Autodesk Inventor part; units mm, degrees
ref_plane "XZ Plane" through (0, 0, 0) normal (0, 1, 0) x (-1, 0, 0)
ref_plane "XY Plane" through (0, 0, 0) normal (0, 0, 1) x (1, 0, 0)
sketch "Sketch1" plane through (0, 0, 0) normal (0, 1, 0) x (-1, 0, 0)
  line L0 (63.5, 50.8) -> (-63.5, 50.8)
  line L1 (-63.5, 50.8) -> (-63.5, -50.8)
  line L2 (-63.5, -50.8) -> (63.5, -50.8)
  line L3 (63.5, -50.8) -> (63.5, 50.8)
  line L4 (63.5, 50.8) -> (-63.5, -50.8) construction
  line L5 (-63.5, 50.8) -> (63.5, -50.8) construction
  point P0 (0, 0)
  dimension "d3" = 101.6
  dimension "d13" = 127
extrude "Extrusion1" add sketch "Sketch1" against normal blind 6.35
sketch "Sketch3" plane through (0, 0, 0) normal (0, 1, 0) x (1, 0, 0)
  line L0 (-63.5, -50.8) -> (-63.5, 50.8) construction
  line L1 (-63.5, -25.4) -> (63.5, -25.4) construction
  line L2 (63.5, 50.8) -> (63.5, -50.8) construction
  line L3 (63.5, 50.8) -> (-63.5, 50.8) construction
  circle A0 centre (-50.8, -25.4) radius 6.35
  circle A1 centre (-25.4, -25.4) radius 6.35
  circle A2 centre (0, -25.4) radius 6.35
  circle A3 centre (25.4, -25.4) radius 6.35
  circle A4 centre (50.8, -25.4) radius 6.35
  point P0 (0, 0)
  dimension "d2" = 76.2
  dimension "d4" = 12.7
  dimension "d5" = 12.7
  dimension "d8" = 25.4
extrude "Extrusion2" cut sketch "Sketch3" against normal through all
properties part number "5-holes"
Geometry check sheet. Reference: the model listing, model coordinates, mm. Give positions to 0.01 mm unless a question says otherwise; leave off trailing zeros. Order: outer loops, then holes, each group sorted by start corner. A loop starts at its lowest first (then second) coordinate and runs counter-clockwise, first axis right, second up.
1) Cross-section at C-C (y = -2.5). Record the boundary of the cut face in (x, z).
Results are:
outline: (-63.5, -50.8) - (63.5, -50.8) - (63.5, 50.8) - (-63.5, 50.8) - close; hole circle Ø12.7 at (-50.8, 25.4); hole circle Ø12.7 at (-25.4, 25.4); hole circle Ø12.7 at (0, 25.4); hole circle Ø12.7 at (25.4, 25.4); hole circle Ø12.7 at (50.8, 25.4)
2) Draft check along Z on faces 1 (the cylindrical face through (56.666, -3.131, 27.832)), 2 (the flat face through (-1, -3, 50.8)), 3 (the flat face through (63.5, -3, 1)). Enter one of: released by +Z, released by -Z, zero draft, split by the parting line, or undercut.
Results are:
face 1: undercut
face 2: released by +Z
face 3: zero draft
3) Cross-section at B-B (x = -50.8). Record the boundary of the cut face in (y, z), then the cut area to 3 significant figures.
Results are:
outline: (-6.35, -50.8) - (0, -50.8) - (0, 19.05) - (-6.35, 19.05) - close; (-6.35, 31.75) - (0, 31.75) - (0, 50.8) - (-6.35, 50.8) - close
area: 565 mm2
4) Gauge pin test, flat end, axial feed: pin 1 (11.5 mm diameter, centred on x = -25.4, z = 25.4, fed in from -Y). Record the tip position at first contact, or that the pin passes through.
Results are:
pin 1: passes through
5) Material ranges on probe 1 along X at (y, z) = (-1.25, 25.4); probe 2 along Z at (x, y) = (50.8, -2); probe 3 along X at (y, z) = (-1.5, 30.5), recorded low to high.
Results are:
probe 1: x = -63.5 to -57.15, -44.45 to -31.75, -19.05 to -6.35, 6.35 to 19.05, 31.75 to 44.45, 57.15 to 63.5
probe 2: z = -50.8 to 19.05, 31.75 to 50.8
probe 3: x = -63.5 to -54.58, -47.02 to -29.18, -21.62 to -3.78, 3.78 to 21.62, 29.18 to 47.02, 54.58 to 63.5
6) Cross-section at A-A (z = 25.4). Record the boundary of the cut face in (x, y).
Results are:
outline: (-63.5, -6.35) - (-57.15, -6.35) - (-57.15, 0) - (-63.5, 0) - close; (-44.45, -6.35) - (-31.75, -6.35) - (-31.75, 0) - (-44.45, 0) - close; (-19.05, -6.35) - (-6.35, -6.35) - (-6.35, 0) - (-19.05, 0) - close; (6.35, -6.35) - (19.05, -6.35) - (19.05, 0) - (6.35, 0) - close; (31.75, -6.35) - (44.45, -6.35) - (44.45, 0) - (31.75, 0) - close; (57.15, -6.35) - (63.5, -6.35) - (63.5, 0) - (57.15, 0) - close
7) Cross-section at D-D (x = -28). Record the boundary of the cut face in (y, z).
Results are:
outline: (-6.35, -50.8) - (0, -50.8) - (0, 19.61) - (-6.35, 19.61) - close; (-6.35, 31.19) - (0, 31.19) - (0, 50.8) - (-6.35, 50.8) - close
